Autodesk Inventor part; units mm, degrees
ref_plane "Work Plane2" through (178, -56.0619, -70.2985) normal (1, 0, 0) x (0, 0.8411785, -0.5407576)
ref_plane "YZ Plane" through (0, 0, 0) normal (1, 0, 0) x (0, 1, 0)
ref_plane "XZ Plane" through (0, 0, 0) normal (0, 1, 0) x (-1, 0, 0)
ref_plane "Work Plane1" through (0, 4.7283, -22.9522) normal (-1, 0, 0) x (0, -0.8411785, 0.5407576)
sketch "Sketch1" plane through (0, 4.7283, -22.9522) normal (-1, 0, 0) x (0, -0.8411785, 0.5407576)
  line L0 (-34.301, -16.75) -> (61.5, -16.75)
  line L1 (61.5, -12.25) -> (61.5, -16.75)
  line L2 (61.5, -16.75) -> (65.5, -16.75)
  line L3 (65.5, -16.75) -> (65.5, -20.25)
  line L4 (65.5, -20.25) -> (79.5, -20.25)
  line L5 (79.5, -20.25) -> (65.5, -11.25)
  line L6 (65.5, -11.25) -> (65.5, -12.25)
  line L7 (65.5, -12.25) -> (61.5, -12.25)
  line L8 (16.3889, 16.75) -> (16.3889, 18.75)
  line L9 (14.3494, 18.75) -> (16.3889, 18.75)
  line L10 (64.2739, -12.25) -> (12.3502, 21.1295)
  line L11 (16.3889, 16.75) -> (16.3889, 18.5332)
  arc A0 (-57.551, -16.75) -> (-61.5, -12.801) centre (-58.75, -14) ccw
  line L12 (-57.551, -16.75) -> (-36.699, -16.75)
  arc A1 (-34.301, -16.75) -> (-36.699, -16.75) centre (-35.5, -14) ccw
  line L13 (-34.301, -16.75) -> (61.5, -16.75)
  line L14 (61.5, -16.75) -> (61.5, -12.25)
  line L15 (61.5, -12.25) -> (16.3889, 16.75)
  line L16 (16.3889, 16.75) -> (-61.5, 16.75)
  line L17 (-61.5, 16.75) -> (-61.5, -12.801)
  line L18 (-61.5, 16.75) -> (-61.5, -12.801)
  arc A2 (-57.551, -16.75) -> (-61.5, -12.801) centre (-58.75, -14) ccw
  line L19 (-57.551, -16.75) -> (-36.699, -16.75)
  arc A3 (-34.301, -16.75) -> (-36.699, -16.75) centre (-35.5, -14) ccw
  line L20 (61.5, -16.75) -> (61.5, -12.25)
  line L21 (61.5, -12.25) -> (16.3889, 16.75)
  line L22 (16.3889, 16.75) -> (-61.5, 16.75)
  point P0 (16.3889, 18.5332)
  point P1 (15.3691, 18.75)
  point P2 (16.3889, 18.5332)
  point P3 (16.0517, 18.75)
  dimension "d14" = 1.5
  dimension "d15" = 2
ref_plane "Work Plane2" through (178, -56.0619, -70.2985) normal (1, 0, 0) x (0, 0.8411785, -0.5407576)
extrude "Extrusion1" add sketch "Sketch1" against normal up to surface (178 mm away) contours L15 L8 L10 L7
sketch "Sketch2" plane through (0, -55.9618, 1.5) normal (0, 0, 1) x (1, 0, 0)
  circle A0 centre (3, 21.9904) radius 2.5
  circle A1 centre (3, 41.3047) radius 2.5
  line L0 (0, 2.3333) -> (0, 55.9618)
  line L1 (0, 2.3333) -> (6, 2.3333)
  line L2 (6, 55.9618) -> (6, 2.3333)
  line L3 (0, 55.9618) -> (6, 55.9618)
  circle A2 centre (175, 21.9904) radius 2.5
  circle A3 centre (175, 41.3047) radius 2.5
  line L4 (178, 2.3333) -> (178, 55.9618)
  line L5 (178, 55.9618) -> (172, 55.9618)
  line L6 (172, 55.9618) -> (172, 2.3333)
  line L7 (178, 2.3333) -> (172, 2.3333)
hole "Hole1" at (3, -14.6571, 1.5) at (3, -33.9713, 1.5) at (175, -33.9713, 1.5) at (175, -14.6571, 1.5) direction (0, 0, -1) diameter 3.6 end through all countersink diameter 7 countersink angle 90
ref_plane "Work Plane3" through (22, -30.5397, -9.0869) normal (0, -0.7712334, 0.6365525) x (1, 0, 0)
sketch "Sketch3" plane through (22, -30.5397, -9.0869) normal (0, -0.7712334, 0.6365525) x (1, 0, 0)
  line L0 (-9.9215, 5.4518) -> (-9.9215, -5.4534)
  spline S0 degree 3 poles (-9.9215, -5.4534) (-9.9222, -5.5772) (-9.8204, -5.8209) (-9.5772, -5.9222) (-9.4534, -5.9215) knots 0 0 0 0 0.5 1 1 1 1
  line L1 (-9.4534, -5.9215) -> (19.4534, -5.9215)
  spline S1 degree 3 poles (19.4534, -5.9215) (19.5775, -5.9222) (19.8219, -5.82) (19.9222, -5.5758) (19.9215, -5.4518) knots 0 0 0 0 0.5 1 1 1 1
  line L2 (19.9215, -5.4518) -> (19.9215, 5.4534)
  spline S2 degree 3 poles (19.9215, 5.4534) (19.9222, 5.5775) (19.82, 5.8219) (19.5758, 5.9222) (19.4518, 5.9215) knots 0 0 0 0 0.5 1 1 1 1
  line L3 (19.4518, 5.9215) -> (-9.4534, 5.9215)
  spline S3 degree 3 poles (-9.4534, 5.9215) (-9.5775, 5.9222) (-9.8219, 5.82) (-9.9222, 5.5758) (-9.9215, 5.4518) knots 0 0 0 0 0.5 1 1 1 1
  circle A0 centre (-8.3791, -4.3791) radius 0.5
  circle A1 centre (-8.3791, 4.3791) radius 0.5
  circle A2 centre (18.3791, 4.3791) radius 0.5
  circle A3 centre (18.3791, -4.3791) radius 0.5
  arc A4 (5.2617, -1.4512) -> (5.1811, -1.5218) centre (5.2771, -1.55) ccw
  arc A5 (5.1811, 1.5218) -> (5.1811, -1.5218) centre (0, 0) ccw
  arc A6 (5.1811, 1.5218) -> (5.2617, 1.4512) centre (5.2771, 1.55) ccw
  arc A7 (5.2617, 1.4512) -> (5.3414, 1.519) centre (5.2463, 1.55) ccw
  arc A8 (5.3414, -1.519) -> (5.3414, 1.519) centre (10, 0) ccw
  arc A9 (5.3414, -1.519) -> (5.2617, -1.4512) centre (5.2463, -1.55) ccw
  line L4 (143.9215, 5.4518) -> (143.9215, -5.4534)
  spline S4 degree 3 poles (143.4534, 5.9215) (143.5775, 5.9222) (143.8219, 5.82) (143.9222, 5.5758) (143.9215, 5.4518) knots 0 0 0 0 0.5 1 1 1 1
  line L5 (114.5482, 5.9215) -> (143.4534, 5.9215)
  spline S5 degree 3 poles (114.0785, 5.4534) (114.0778, 5.5775) (114.18, 5.8219) (114.4242, 5.9222) (114.5482, 5.9215) knots 0 0 0 0 0.5 1 1 1 1
  line L6 (114.0785, -5.4518) -> (114.0785, 5.4534)
  spline S6 degree 3 poles (114.5466, -5.9215) (114.4225, -5.9222) (114.1781, -5.82) (114.0778, -5.5758) (114.0785, -5.4518) knots 0 0 0 0 0.5 1 1 1 1
  line L7 (143.4534, -5.9215) -> (114.5466, -5.9215)
  spline S7 degree 3 poles (143.9215, -5.4534) (143.9222, -5.5772) (143.8204, -5.8209) (143.5772, -5.9222) (143.4534, -5.9215) knots 0 0 0 0 0.5 1 1 1 1
  circle A10 centre (142.3791, -4.3791) radius 0.5
  circle A11 centre (142.3791, 4.3791) radius 0.5
  circle A12 centre (115.6209, 4.3791) radius 0.5
  circle A13 centre (115.6209, -4.3791) radius 0.5
  arc A14 (128.8189, -1.5218) -> (128.7383, -1.4512) centre (128.7229, -1.55) ccw
  arc A15 (128.7383, -1.4512) -> (128.6586, -1.519) centre (128.7537, -1.55) ccw
  arc A16 (128.6586, 1.519) -> (128.6586, -1.519) centre (124, 0) ccw
  arc A17 (128.6586, 1.519) -> (128.7383, 1.4512) centre (128.7537, 1.55) ccw
  arc A18 (128.7383, 1.4512) -> (128.8189, 1.5218) centre (128.7229, 1.55) ccw
  arc A19 (128.8189, -1.5218) -> (128.8189, 1.5218) centre (134, 0) ccw
  circle A20 centre (10, 0) radius 5.4
  circle A21 centre (124, 0) radius 5.4
  line L8 (0, 5.4) -> (10, 5.4)
  line L9 (10, -5.4) -> (0, -5.4)
  line L10 (124, 5.4) -> (134, 5.4)
  line L11 (134, -5.4) -> (124, -5.4)
  point P0 (-22, 26.4483)
  dimension "d9" = 10.8
  dimension "d10" = 10.8
extrude "Extrusion2" cut sketch "Sketch3" along normal blind 78.25 contours A9 A8 A7 A6 A5 A20 A4 | A4 A5 A20 A6 A7 A8 A9 | A20 L9 A5 | A5 A20 | A5 L8 A20 | A19 A21 A18 A17 A16 A15 A14 | A14 A15 A16 A17 A18 A19 A21 | A21 A19 | A19 L11 A21 | A19 A21 L10
properties part number "front" material "Aluminum 6061"
Work out the finished part from the listing and answer in its coordinate system (mm). A direction names the side the tool comes from. Coordinates: 2 decimals unless noted, no trailing zeros. Loops run counter-clockwise (first coordinate to the right, second up) from the corner with the lowest first, then second, coordinate; pieces in that order, holes last.
1) For a pull along Y with two mould halves and no side action, classify faces 3 (the conical face through (172.793, -14.167, 0.26)), 4 (the flat face through (88, -27, 0)) as +Y half, -Y half, draft (parallel to the pull), parting line (faces both ways), or undercut.
Results:
face 3: undercut
face 4: draft
2) Consider probe 1 along X at (y, z) = (-43.5, 1.15); probe 2 along X at (y, z) = (-48.5, 1); probe 3 along Y at (x, z) = (157.5, 0.45). Determine where each line is inside the solid, lowest interval first.
Results:
probe 1: x = 0 to 16.61, 37.39 to 140.61, 161.39 to 178
probe 2: x = 0 to 18.02, 35.98 to 142.02, 159.98 to 178
probe 3: y = -54.33 to -50.24, -33.95 to 0.29
3) Section C-C (y = -47) is taken. Give the number of separate pieces and of enclosed holes in the cut face, plus the area to 3 significant figures.
Results:
separate pieces: 3
enclosed holes: 0
area: 210 mm2
4) Section A-A (x = 175) is taken. Give the vertices of the cut face in (y, z).
Results:
outline: (-55.96, 1.5) - (-53.63, 0) - (-35.97, 0) - (-37.47, 1.5) - close; (-31.97, 0) - (-16.66, 0) - (-18.16, 1.5) - (-30.47, 1.5) - close; (-12.66, 0) - (0, 0) - (0.96, 1.5) - (-11.16, 1.5) - close
5) For faces 1 (the cylindrical face through (140.6, -42.5, 0.7)), 2 (the conical face through (5.24, -14.36, 0.26)), determine the directions among +Z, -Z, +X, -X, +Y, -Y from which every point of the face is accessible in a straight line to the end or side of a thin tool.
Results:
face 1: none
face 2: +Z
6) Section B-B (x = 70.5) is taken. Give the vertices of the cut face in (y, z), plus the area to 3 significant figures.
Results:
outline: (-55.96, 1.5) - (-53.63, 0) - (0, 0) - (0.96, 1.5) - close
area: 82.9 mm2
